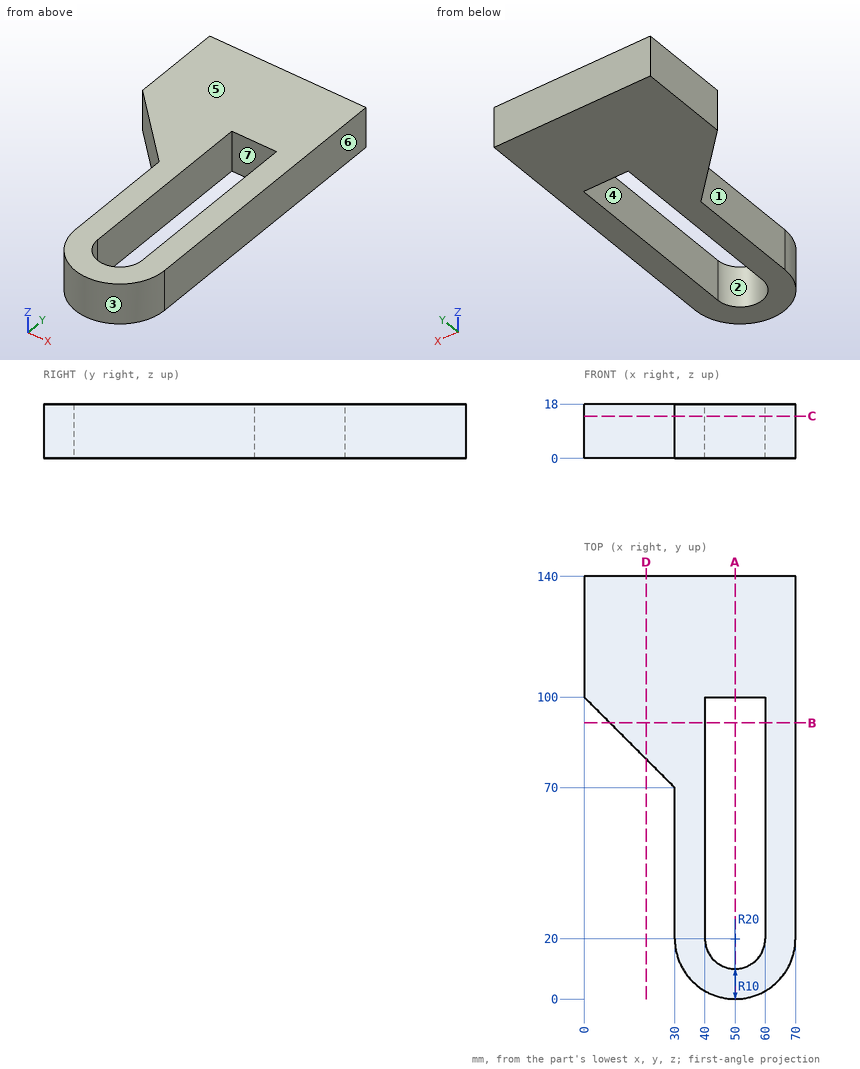
Print and shaded views of the part. All mm, measured from the part's lowest x, y and z. A direction names the side the tool comes from. Round coordinates to 2 decimals unless told otherwise and drop trailing zeros. Write each loop counter-clockwise with the first axis right and the second up, starting at its lowest first coordinate (ties: lowest second). Pieces come first, ordered by that corner, then holes. Notation, with made-up numbers: (68, 87) - (90, 87) arc R15 ccw to (90, 92) - close; hole circle Ø6 at (-27.5, 76.25). An arc over 180 degrees is marked (long way). One line per question, with ' | ' between items.
1. Drop flat-ended pins along their axis: pin 1 Ø8 at (x, z) = (11.5, 16) entering from -Y; pin 2 Ø6 at (y, z) = (32.5, 13) entering from -X. Give the stop position or say it passes through.
Results are:
pin 1: y = 84.5 | pin 2: x = 30
2. Band-saw the part on A-A, the plane x = 50. Write the cut outline in (y, z).
Results are:
outline: (0, 0) - (10, 0) - (10, 18) - (0, 18) - close; (100, 0) - (140, 0) - (140, 18) - (100, 18) - close
3. Tool access for the marked faces 1, 2 and 3: list every direction of +Z, -Z, +X, -X, +Y, -Y with a clear straight run to the whole face (end or side of a thin tool).
Results are:
face 1: +Z, -Z, -X, -Y | face 2: +Z, -Z | face 3: +Z, -Z, -Y
4. Band-saw the part on B-B, the plane y = 91.5. Write the cut outline in (x, z).
Results are:
outline: (8.5, 0) - (40, 0) - (40, 18) - (8.5, 18) - close; (60, 0) - (70, 0) - (70, 18) - (60, 18) - close
5. Drill centre lines: line 1 along X through (y, z) = (35, 11); line 2 along Y through (x, z) = (44, 4.25); line 3 along X through (y, z) = (17.5, 10.25). Where is each one in solid material? Low to high. Write a range as from..to.
Results are:
line 1: 30..40, 60..70 | line 2: 0.92..12, 100..140 | line 3: 30.16..40.32, 59.68..69.84
6. Mould opens along X. For the marked faces 4, 5, 6 and 7 say: released by +X, released by -X, zero draft, split by the parting line, or undercut.
Results are:
face 4: undercut | face 5: zero draft | face 6: released by +X | face 7: undercut
7. Band-saw the part on C-C, the plane z = 14. Write the cut outline in (x, y), and give its area (3 significant figures).
Results are:
outline: (0, 100) - (30, 70) - (30, 20) arc R20 ccw to (70, 20) - (70, 140) - (0, 140) - close; hole (40, 20) arc R10 ccw to (60, 20) - (60, 100) - (40, 100) - close | area: 5,320 mm^2
8. Band-saw the part on D-D, the plane x = 20.5. Write the cut outline in (y, z), and give its area (3 significant figures).
Results are:
outline: (79.5, 0) - (140, 0) - (140, 18) - (79.5, 18) - close | area: 1,090 mm^2
